```python
from build123d import *

# Parameters (mm, degrees)
F1_DEPTH    = 19.05
F2_T1_DEPTH = 82.895018686
F3_R        = 7.61999
F5_W        = 2.54
F5_H        = 1.27
F6_DEPTH    = 3.81
F4_W        = 5.08
F4_H        = 2.54
F7_DEPTH    = 1.27
F8_R        = 1.26999


# Not quite as in the source:
# - a fillet or chamfer that OpenCascade refuses, or shapes differently, is made with other operations: its cross-section is extruded or revolved along the edge and cut away or added
# - a fillet or chamfer is up to 0.001 mm smaller than in the source, because OpenCascade refuses the exact size


with BuildPart() as f1:
    # F0 (on Right) → F1 (new body)
    with BuildSketch(Plane.YZ):
        Polygon((-22.9305560945, 20.32), (0, 0), (65.9694439055, 0), (65.9694439055, 12.7), (8.8194439055, 12.7), (8.8194439055, 20.32), align=None)
    extrude(amount=F1_DEPTH)

    # F2: chamfer of 10.16 on 2 edges, made by hand

    # F2_s2 → F2_t1 (cut)
    with BuildSketch(Plane(origin=(0, -42.4856252608, 37.6487993462), x_dir=(1, 0, 0), z_dir=(0, 0.7484248802, -0.6632195705))):
        Polygon((8.89, 0), (19.05, -10.16), (19.05, 0), align=None)
        Polygon((10.16, 0), (0, -10.16), (0, 0), align=None)
    extrude(amount=F2_T1_DEPTH, mode=Mode.SUBTRACT)

    # F3 (radius 7.62 in the source; OpenCascade refuses exactly that, so slightly less here)
    f3_edges = [f1.edges().sort_by_distance(p)[0] for p in [
        (0, 3.853932, 10.16),
        (0, 40.644327, 0),
        (19.05, 40.644327, 0),
        (19.05, 3.853932, 10.16),
        (9.525, 8.819444, 12.7),
    ]]
    fillet(f3_edges, radius=F3_R)

    # F5 (on face) → F6 (join)
    with BuildSketch(Plane.XY.offset(12.7)):
        with Locations((9.525, 17.7094439055)):
            Rectangle(F5_W, F5_H)
        with Locations((9.525, 64.6994439055)):
            Rectangle(F5_W, F5_H)
    extrude(amount=F6_DEPTH)

    # F4 (on face) → F7 (join)
    with BuildSketch(Plane.XY.offset(12.7)):
        with Locations((9.525, 17.7094439055)):
            Rectangle(F4_W, F4_H)
        with Locations((9.525, 64.6994439055)):
            Rectangle(F4_W, F4_H)
    extrude(amount=F7_DEPTH)

    # F8 (radius 1.27 in the source; OpenCascade refuses exactly that, so slightly less here)
    f8_edges = [f1.edges().sort_by_distance(p)[0] for p in [
        (10.795, 17.709444, 16.51),
        (8.255, 17.709444, 16.51),
        (8.255, 64.699444, 16.51),
        (10.795, 64.699444, 16.51),
    ]]
    fillet(f8_edges, radius=F8_R)


solid = f1.part
```
For this review, take the finished solid that the model builds, in its own axes (mm). A direction names the side the tool comes from. Round coordinates to 2 decimals unless told otherwise and drop trailing zeros. Order: outer loops, then holes, each group sorted by start corner. A loop starts at its lowest first (then second) coordinate and runs counter-clockwise, first axis right, second up.
Q1. Insertion check: P1, Ø1.5, axis at x = 3.5, z = 4.5, coming from the -Y side; P2, Ø0.8, axis at x = 10, z = 15, coming from the +Y side; P3, Ø0.6, axis at y = 65, z = 14.5, coming from the +X side (3 decimals). Each pin has a flat end and moves straight along its axis. Give the tip position at first contact, or say it passes through.
Findings below:
P1: stops at y = 3.55
P2: stops at y = 65.33
P3: stops at x = 10.795
Q2. Wall thickness on line 1 (Y direction, x = 8.5, z = 14.5); line 2 (Z direction, x = 12.5, y = -13.5); line 3 (X direction, y = -3, z = 12.25): over which ranges is each line inside the solid? List them lowest first.
Findings below:
line 1: y = -13.86 to 11.52, 17.07 to 18.34, 64.06 to 65.33
line 2: z = 16.79 to 20.32
line 3: x = 2.98 to 16.07
Q3. We need section A-A, the plane y = 44.5. Give the boundary of the cut face in (x, z), plus the area to 3 significant figures.
Findings below:
outline: (0, 7.62) arc R7.62 ccw to (7.62, 0) - (11.43, 0) arc R7.62 ccw to (19.05, 7.62) - (19.05, 12.7) - (0, 12.7) - close
area: 217 mm2
Q4. Machinability: for faces 4 (the flat face through (10, 18.344, 15)), 5 (the flat face through (5.93, -6.43, 11.35)), 6 (the flat face through (10, 65.334, 15)), which of the approach directions +Z, -Z, +X, -X, +Y, -Y give a long, thin tool a straight path to every point of the face, cutting with its end or side? Answer none if there is none.
Findings below:
face 4: +Z, +X, -X
face 5: -Z, -X, -Y
face 6: +Z, +X, -X, +Y
Q5. Mouldability with a two-part tool opening along Y and no side actions: class faces 1 (the cylindrical face through (18.454, 0.986, 12.971)), 2 (the flat face through (9, 42, 12.7)), 3 (the flat face through (0, 31, 11)) as pulls with the +Y half, pulls with the -Y half, needs draft (parallel to the pull), parting line crosses it, or undercut.
Findings below:
face 1: pulls with the -Y half
face 2: undercut
face 3: needs draft
Q6. We need section D-D, the plane y = 14. Give the boundary of the cut face in (x, z), plus the area to 3 significant figures.
Findings below:
outline: (0, 7.62) arc R7.62 ccw to (7.62, 0) - (11.43, 0) arc R7.62 ccw to (19.05, 7.62) - (19.05, 13.1) - (0, 13.1) - close
area: 225 mm2
